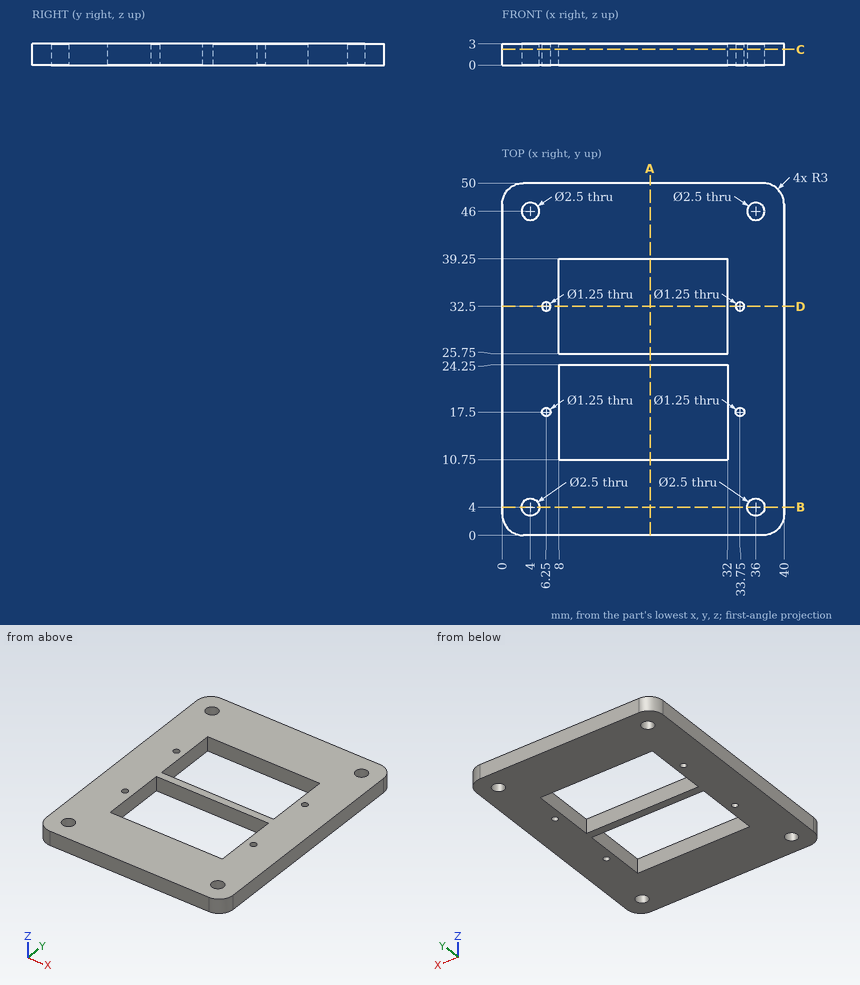
Geometry: see drawing. Coordinates: mm, zero at the bounding-box minimum. Give positions to 0.01 mm unless a question says otherwise; leave off trailing zeros. Loops run counter-clockwise (first coordinate to the right, second up) from the corner with the lowest first, then second, coordinate; pieces in that order, holes last. Notation, with made-up numbers: M 17,21 L 51,21 A18 ccw 51,40 Z; hole C 47.25,78 d3. An arc over 180 degrees is marked long. Use one line per item in the form item = value.
1. Section query C-C, the plane z = 2.25. Count the separate pieces of the cut face and the enclosed holes in it, and give its area (3 significant figures).
Numbers:
separate_pieces = 1
enclosed_holes = 10
area = 1,320 mm²
2. Line query: L1, parallel to Y at x = 9.5, z = 2.25; L2, parallel to X at y = 4, z = 1.75; L3, parallel to X at y = 32.5, z = 1.8 (3 decimals). Output: solid intervals per line, ascending.
Numbers:
L1 = 0 to 10.75, 24.25 to 25.75, 39.25 to 50
L2 = 0 to 2.75, 5.25 to 34.75, 37.25 to 40
L3 = 0 to 5.625, 6.875 to 8, 32 to 33.125, 34.375 to 40
3. Section query A-A, the plane x = 21. Return the cut outline in (y, z), and give its area (3 significant figures).
Numbers:
outline = M 0,0 L 10.75,0 L 10.75,3 L 0,3 Z; M 24.25,0 L 25.75,0 L 25.75,3 L 24.25,3 Z; M 39.25,0 L 50,0 L 50,3 L 39.25,3 Z
area = 69.0 mm²
4. Section query D-D, the plane y = 32.5. Return the cut outline in (x, z) (3 decimals), and give its area (3 significant figures).
Numbers:
outline = M 0,0 L 5.625,0 L 5.625,3 L 0,3 Z; M 6.875,0 L 8,0 L 8,3 L 6.875,3 Z; M 32,0 L 33.125,0 L 33.125,3 L 32,3 Z; M 34.375,0 L 40,0 L 40,3 L 34.375,3 Z
area = 40.5 mm²
5. Section query B-B, the plane y = 4. Return the cut outline in (x, z).
Numbers:
outline = M 0,0 L 2.75,0 L 2.75,3 L 0,3 Z; M 5.25,0 L 34.75,0 L 34.75,3 L 5.25,3 Z; M 37.25,0 L 40,0 L 40,3 L 37.25,3 Z
